Model file for the job. Use its own axes, mm. A direction names the side the tool comes from. Coordinates: 2 decimals unless noted, no trailing zeros. Write each loop counter-clockwise with the first axis right and the second up, starting at its lowest first coordinate (ties: lowest second). Pieces come first, ordered by that corner, then holes. Notation, with made-up numbers: (32, 37.25) - (51, 37.25) arc R31 cw to (51, 74.25) - close; hole circle Ø11 at (19, 62.5). An arc over 180 degrees is marked (long way). Put each result on its own line as item: value. Start each with the question number.
1. Saw through at A-A, the plane y = 11. Give the number of separate pieces and of enclosed holes in the cut face, plus the area to 3 significant figures.
2. Saw through at B-B, the plane z = -137.5. Write the cut outline in (x, y), plus the area to 3 significant figures.
3. Drill centre lines: L1, parallel to Z at x = 3, y = 23.5; L2, parallel to Z at x = 143, y = 5.5; L3, parallel to X at y = 32, z = -95. Where is each one in solid material? Low to high. Write a range as from..to.
4. Pull direction X, two halves, no side cores. Call faces 1 (the face through (47, -5, -287.434)), 2 (the face through (125.8, 37, 51)), 3 (the face through (26.564, 36, 222)): released by +X, released by -X, zero draft, split by the parting line, or undercut.
5. Drop flat-ended pins along their axis: P1, Ø1.5, axis at x = 60.5, y = 60.5, coming from the -Z side; P2, Ø1, axis at x = 40, y = 44.5, coming from the +Z side; P3, Ø4, axis at x = -51, y = 51, coming from the +Z side; P4, Ø2, axis at y = 42, z = -38.5, coming from the -X side. Give the stop position or say it passes through.
6. Which spindle directions (+Z, -Z, +X, -X, +Y, -Y) get a long thin tool onto all of the face, cutting with end or side? Do faces 4 (the face through (152, 36, 108.988)), 5 (the face through (0, 20, -50)), 6 (the face through (161.915, 55.37, 108.462)). Say none if no direction does.
7. Saw through at C-C, the plane x = 150. Write the cut outline in (y, z), plus the area to 3 significant figures.
```python
from build123d import *

# Parameters (mm, degrees)
SKETCH1_W             = 101.6
SKETCH1_H             = 101.6
BOSS_EXTRUDE1_DEPTH   = 39.99992
SKETCH2_W             = 98.115054024
SKETCH2_H             = 98.519374302
CUT_EXTRUDE1_DEPTH    = 35.56
SKETCH3_W             = 49.9999
SKETCH3_H             = 37.999924
BOSS_EXTRUDE2_DEPTH   = 75.000104
SKETCH3_W_2           = 50.038
SKETCH3_H_2           = 38.1
BOSS_EXTRUDE2_2_DEPTH = 75.000104
BOSS_EXTRUDE2_3_DEPTH = 75.000104
BOSS_EXTRUDE2_4_DEPTH = 75.000104
SKETCH3_W_3           = 50.044709845
SKETCH3_H_3           = 38.200481576
BOSS_EXTRUDE2_5_DEPTH = 75.000104
SKETCH4_W             = 47.673303357
SKETCH4_H             = 36.001078641
SKETCH4_W_2           = 47.329126014
SKETCH4_H_2           = 35.49131434
SKETCH4_W_3           = 47.385353059
SKETCH4_H_3           = 34.904518915
SKETCH4_W_4           = 47.458878428
SKETCH4_W_5           = 48.104938799
SKETCH4_H_4           = 35.956464733
CUT_EXTRUDE2_DEPTH    = 73.222104
SKETCH5_R             = 9.906
SKETCH5_R_2           = 9.962701018
CUT_EXTRUDE3_DEPTH    = 9.722104
SKETCH6_R             = 9.906
CUT_EXTRUDE4_DEPTH    = 9.722104
SKETCH7_R             = 9.906
CUT_EXTRUDE5_DEPTH    = 9.722104
SKETCH8_W             = 297.716106252
SKETCH8_H             = 549.396882706
BOSS_EXTRUDE4_DEPTH   = 9.722104
SKETCH9_R             = 3.175
BOSS_EXTRUDE5_DEPTH   = 25.4


with BuildPart() as part:
    # Sketch1 → Boss-Extrude1 (new body)
    with BuildSketch(Plane(origin=(0, 0, 0), x_dir=(1, 0, 0), z_dir=(0, 1, 0))):
        with Locations((50.8, 50.8)):
            Rectangle(SKETCH1_W, SKETCH1_H)
    extrude(amount=BOSS_EXTRUDE1_DEPTH)

    # Sketch2 → Cut-Extrude1 (cut)
    with BuildSketch(Plane(origin=(0, 39.99992, 0), x_dir=(1, 0, 0), z_dir=(0, 1, 0))):
        with Locations((50.665226574, 50.597839861)):
            Rectangle(SKETCH2_W, SKETCH2_H)
    extrude(amount=-CUT_EXTRUDE1_DEPTH, mode=Mode.SUBTRACT)



with BuildPart() as body_2:
    # Sketch3 → Boss-Extrude2 (new body)
    with BuildSketch(Plane.XZ):
        with Locations((100.7999508, 50.8000254)):
            Rectangle(SKETCH3_W, SKETCH3_H)
    extrude(amount=-BOSS_EXTRUDE2_DEPTH)


with BuildPart() as body_3:
    # Sketch3 → Boss-Extrude2 2 (new body)
    with BuildSketch(Plane.XZ):
        with Locations((0.7809992, 50.7499874)):
            Rectangle(SKETCH3_W_2, SKETCH3_H_2)
    extrude(amount=-BOSS_EXTRUDE2_2_DEPTH)


with BuildPart() as body_4:
    # Sketch3 → Boss-Extrude2 3 (new body)
    with BuildSketch(Plane.XZ):
        with Locations((152.019, 127)):
            Rectangle(SKETCH3_W_2, SKETCH3_H_2)
    extrude(amount=-BOSS_EXTRUDE2_3_DEPTH)


with BuildPart() as body_5:
    # Sketch3 → Boss-Extrude2 4 (new body)
    with BuildSketch(Plane.XZ):
        with Locations((-50.419, 127)):
            Rectangle(SKETCH3_W_2, SKETCH3_H_2)
    extrude(amount=-BOSS_EXTRUDE2_4_DEPTH)


with BuildPart() as body_6:
    # Sketch3 → Boss-Extrude2 5 (new body)
    with BuildSketch(Plane.XZ):
        with Locations((50.669645078, 222.300240788)):
            Rectangle(SKETCH3_W_3, SKETCH3_H_3)
    extrude(amount=-BOSS_EXTRUDE2_5_DEPTH)


with BuildPart() as cut_extrude2_tool:
    # Sketch4 → Cut-Extrude2 (new body)
    with BuildSketch(Plane.XZ):
        with Locations((-50.459366902, 126.988435685)):
            Rectangle(SKETCH4_W, SKETCH4_H)
        with Locations((0.970104392, 50.412109166)):
            Rectangle(SKETCH4_W_2, SKETCH4_H_2)
        with Locations((100.689433749, 50.705506879)):
            Rectangle(SKETCH4_W_3, SKETCH4_H_3)
        with Locations((152.233471247, 126.988435685)):
            Rectangle(SKETCH4_W_4, SKETCH4_H)
        with Locations((50.616530906, 222.262061552)):
            Rectangle(SKETCH4_W_5, SKETCH4_H_4)
    extrude(amount=-CUT_EXTRUDE2_DEPTH)


with BuildPart() as body_2_1:
    add(body_2.part)

    # Cut-Extrude2: cut by cut_extrude2_tool
    add(cut_extrude2_tool.part, mode=Mode.SUBTRACT)


with BuildPart() as body_3_1:
    add(body_3.part)

    # Cut-Extrude2: cut by cut_extrude2_tool
    add(cut_extrude2_tool.part, mode=Mode.SUBTRACT)


with BuildPart() as body_4_1:
    add(body_4.part)

    # Cut-Extrude2: cut by cut_extrude2_tool
    add(cut_extrude2_tool.part, mode=Mode.SUBTRACT)


with BuildPart() as body_5_1:
    add(body_5.part)

    # Cut-Extrude2: cut by cut_extrude2_tool
    add(cut_extrude2_tool.part, mode=Mode.SUBTRACT)


with BuildPart() as body_6_1:
    add(body_6.part)

    # Cut-Extrude2: cut by cut_extrude2_tool
    add(cut_extrude2_tool.part, mode=Mode.SUBTRACT)

    # Sketch7 → Cut-Extrude5 (cut)
    with BuildSketch(Plane(origin=(0, 0, 203.2), x_dir=(-1, 0, 0), z_dir=(0, 0, -1))):
        with Locations((-50.669645078, 54.934104)):
            Circle(SKETCH7_R)
    extrude(amount=-CUT_EXTRUDE5_DEPTH, mode=Mode.SUBTRACT)


with BuildPart() as cut_extrude3_tool:
    # Sketch5 → Cut-Extrude3 (new body)
    with BuildSketch(Plane(origin=(0, 0, 31.6999874), x_dir=(-1, 0, 0), z_dir=(0, 0, -1))):
        with Locations((-0.7809992, 54.934104)):
            Circle(SKETCH5_R)
        with Locations((-100.7999508, 54.934104)):
            Circle(SKETCH5_R_2)
    extrude(amount=-CUT_EXTRUDE3_DEPTH)


with BuildPart() as body_2_2:
    add(body_2_1.part)

    # Cut-Extrude3: cut by cut_extrude3_tool
    add(cut_extrude3_tool.part, mode=Mode.SUBTRACT)


with BuildPart() as body_3_2:
    add(body_3_1.part)

    # Cut-Extrude3: cut by cut_extrude3_tool
    add(cut_extrude3_tool.part, mode=Mode.SUBTRACT)


with BuildPart() as cut_extrude4_tool:
    # Sketch6 → Cut-Extrude4 (new body)
    with BuildSketch(Plane(origin=(0, 0, 107.95), x_dir=(-1, 0, 0), z_dir=(0, 0, -1))):
        with Locations((-152.019, 54.934104)):
            Circle(SKETCH6_R)
        with Locations((50.419, 54.934104)):
            Circle(SKETCH6_R)
    extrude(amount=-CUT_EXTRUDE4_DEPTH)


with BuildPart() as body_4_2:
    add(body_4_1.part)

    # Cut-Extrude4: cut by cut_extrude4_tool
    add(cut_extrude4_tool.part, mode=Mode.SUBTRACT)


with BuildPart() as body_5_2:
    add(body_5_1.part)

    # Cut-Extrude4: cut by cut_extrude4_tool
    add(cut_extrude4_tool.part, mode=Mode.SUBTRACT)


with BuildPart() as part_1:
    add(part.part)

    add(body_2_2.part)  # Boss-Extrude4 merges body 2

    add(body_3_2.part)  # Boss-Extrude4 merges body 3

    add(body_4_2.part)  # Boss-Extrude4 merges body 4

    add(body_5_2.part)  # Boss-Extrude4 merges body 5

    add(body_6_1.part)  # Boss-Extrude4 merges body 6
    # Sketch8 → Boss-Extrude4 (add)
    with BuildSketch(Plane.XZ):
        with Locations((49.547758626, -12.735627368)):
            Rectangle(SKETCH8_W, SKETCH8_H)
    extrude(amount=BOSS_EXTRUDE4_DEPTH)

    # Sketch9 → Boss-Extrude5 (add)
    with BuildSketch(Plane(origin=(0, 0, 0), x_dir=(1, 0, 0), z_dir=(0, 1, 0))):
        with Locations(Location((25.4, 152.4, 0), (0, 0, 90))):
            Circle(SKETCH9_R)
        with Locations(Location((76.2, 152.4, 0), (0, 0, 90))):
            Circle(SKETCH9_R)
    extrude(amount=BOSS_EXTRUDE5_DEPTH)


solid = part_1.part
```
Final values:
1. separate pieces: 8
1. enclosed holes: 6
1. area: 1,760 mm²
2. outline: (-99.31, -9.72) - (198.41, -9.72) - (198.41, 0) - (-99.31, 0) - close
2. area: 2,890 mm²
3. L1: z = -101.6..-99.86, -1.34..0, 31.7..32.67, 68.16..69.8
3. L2: z = 107.95..108.99, 144.99..146.05
3. L3: x = 0..1.61, 99.72..101.6
4. face 1: zero draft
4. face 2: released by +X
4. face 3: undercut
5. P1: stops at z = 203.2
5. P2: stops at z = 241.4
5. P3: stops at z = 146.05
5. P4: passes through
6. face 4: none
6. face 5: -Z, -X, +Y
6. face 6: -Z
7. outline: (-9.72, -287.43) - (0, -287.43) - (0, 107.95) - (45.24, 107.95) - (45.24, 108.99) - (0, 108.99) - (0, 144.99) - (73.22, 144.99) - (73.22, 108.99) - (64.63, 108.99) - (64.63, 107.95) - (75, 107.95) - (75, 146.05) - (0, 146.05) - (0, 261.96) - (-9.72, 261.96) - close
7. area: 5,540 mm²
